from build123d import *

# Parameters (mm, degrees)
F0_W     = 1450
F0_H     = 415
F1_DEPTH = 20
F2_W     = 20
F2_H     = 13
F3_DEPTH = 1450
F5_DEPTH = 510
F6_W     = 1450
F6_H     = 25
F7_DEPTH = 25


with BuildPart() as f1:
    # F0 (on Top) → F1 (new body)
    with BuildSketch(Plane.XY):
        Rectangle(F0_W, F0_H)
    extrude(amount=F1_DEPTH)

    # F2 (on face) → F3 (cut)
    with BuildSketch(Plane.YZ.offset(725)):
        with Locations((197.5, 13.5)):
            Rectangle(F2_W, F2_H)
    extrude(amount=-F3_DEPTH, mode=Mode.SUBTRACT)

    # F4 (on face) → F5 (cut)
    with BuildSketch(Plane.XZ.offset(207.5)):
        Polygon((725, 0), (725, 20), (705, 20), align=None)
        Polygon((-725, 20), (-725, 0), (-705, 20), align=None)
    extrude(amount=-F5_DEPTH, mode=Mode.SUBTRACT)

    # F6 (on face) → F7 (cut)
    with BuildSketch(Plane(origin=(0, 0, 0), x_dir=(1, 0, 0), z_dir=(0, 0, -1))):
        with Locations((0, 195)):
            Rectangle(F6_W, F6_H)
    extrude(amount=-F7_DEPTH, mode=Mode.SUBTRACT)


solid = f1.part
Can you work these out from the model? Positions are in its coordinate system, mm. Coordinates: 2 decimals unless noted, no trailing zeros. Order: outer loops, then holes, each group sorted by start corner. A loop starts at its lowest first (then second) coordinate and runs counter-clockwise, first axis right, second up. Notation, with made-up numbers: M 23.5,84 L 34.5,84 A27 cw 34.5,115 Z; hole C 45.5,23.25 d6. An arc over 180 degrees is marked long. Answer as CSV lines item,"result".
(1) Suppose I cut it at A-A on z = 15.75. Please give me the cut outline in (x, y).
Geometry check:
outline,"M -709.25,-182.5 L 709.25,-182.5 L 709.25,187.5 L -709.25,187.5 Z"
(2) Suppose I cut it at B-B on x = -49. Please give me the cut outline in (y, z), plus the area to 3 significant figures.
Geometry check:
outline,"M -182.5,0 L 207.5,0 L 207.5,7 L 187.5,7 L 187.5,20 L -182.5,20 Z"
area,"7,540 mm^2"
(3) Please list where these lines run through material, in increasing order: L1, parallel to Z at x = 423.5, y = 190.5; L2, parallel to Y at x = 227, z = 16; L3, parallel to X at y = 64, z = 7.
Geometry check:
L1,"0 to 7"
L2,"-182.5 to 187.5"
L3,"-718 to 718"
(4) I'm going to push flat-ended pins straight in: pin 1 (5 mm diameter, centred on y = -35.5, z = 7, fed in from +X); pin 2 (3 mm diameter, centred on y = -121.5, z = 7, fed in from -X); pin 3 (6 mm diameter, centred on x = -280.5, y = 202.5, fed in from +Z). Where does each tip first touch, or does it pass through?
Geometry check:
pin 1,"x = 720.5"
pin 2,"x = -719.5"
pin 3,"z = 7"
